Input: part model. Units: mm. Frame: model coordinates. Face numbers are marked on the shaded views. A direction names the side the tool comes from. Give positions to 0.01 mm unless a question says otherwise; leave off trailing zeros. Loops run counter-clockwise (first coordinate to the right, second up) from the corner with the lowest first, then second, coordinate; pieces in that order, holes last.
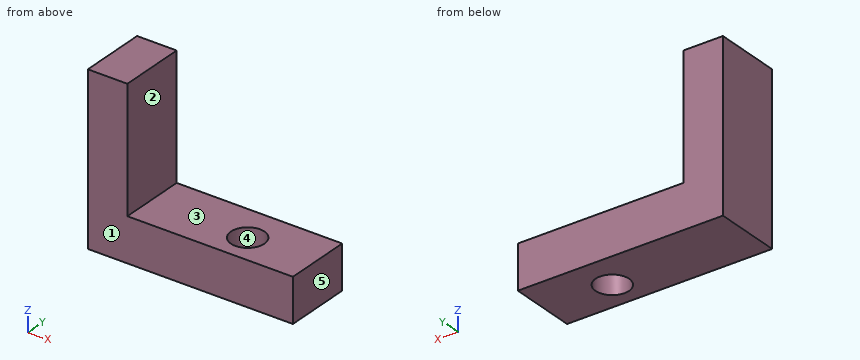
from build123d import *

# Parameters (mm, degrees)
F1_DEPTH = 25.4
F2_R     = 6.35
F3_DEPTH = 25.4


with BuildPart() as f1:
    # F0 (on Front) → F1 (new body)
    with BuildSketch(Plane.XZ):
        Polygon((-28.737951, 39.518028), (-43.749195, 39.518028), (-43.749195, -23.760144), (-28.737951, -23.760144), (34.078334, -23.760144), (34.078334, -7.132303), (-28.737951, -7.132303), align=None)
    extrude(amount=F1_DEPTH)

    # F2 (on face) → F3 (cut)
    with BuildSketch(Plane.XY.offset(-7.132303)):
        with Locations((8.678334, -14.20567)):
            Circle(F2_R)
    extrude(amount=-F3_DEPTH, mode=Mode.SUBTRACT)


solid = f1.part
(1) Ray query, probe 1 along X at (y, z) = (-23.5, -1); probe 2 along X at (y, z) = (-16, -19); probe 3 along Z at (x, y) = (-28, -21). Return the intervals inside material, ascending.
Values follow:
probe 1: x = -43.75 to -28.74
probe 2: x = -43.75 to 2.59, 14.77 to 34.08
probe 3: z = -23.76 to -7.13
(2) Cut plane D-D (y = -3.25). Return the cut outline in (x, z).
Values follow:
outline: (-43.75, -23.76) - (34.08, -23.76) - (34.08, -7.13) - (-28.74, -7.13) - (-28.74, 39.52) - (-43.75, 39.52) - close
(3) Cut plane A-A (y = -9.5). Return the cut outline in (x, z), and give its area (3 significant figures).
Values follow:
outline: (-43.75, -23.76) - (4.41, -23.76) - (4.41, -7.13) - (-28.74, -7.13) - (-28.74, 39.52) - (-43.75, 39.52) - close; (12.94, -23.76) - (34.08, -23.76) - (34.08, -7.13) - (12.94, -7.13) - close
area: 1,850 mm2
(4) Reachability of the marked faces 1 and 2 from +Z, -Z, +X, -X, +Y, -Y: full face, straight path, thin tool, end or side. Return the list, or none.
Values follow:
face 1: +Z, -Z, +X, -X, -Y
face 2: +Z, +X, +Y, -Y
(5) Pin query (flat end, axial travel): pin 1 Ø12.5 at (y, z) = (-13.5, 7) entering from +X; pin 2 Ø1.5 at (x, y) = (2, -4) entering from +Z. Return the tip coordinate at first contact, or that it passes through.
Values follow:
pin 1: stops at x = -28.74
pin 2: stops at z = -7.13
(6) Cut plane B-B (x = 12.5). Return the cut outline in (y, z), and give its area (3 significant figures).
Values follow:
outline: (-25.4, -23.76) - (-19.28, -23.76) - (-19.28, -7.13) - (-25.4, -7.13) - close; (-9.13, -23.76) - (0, -23.76) - (0, -7.13) - (-9.13, -7.13) - close
area: 254 mm2
(7) Cut plane C-C (z = -15). Return the cut outline in (x, y), and give its area (3 significant figures).
Values follow:
outline: (-43.75, -25.4) - (34.08, -25.4) - (34.08, 0) - (-43.75, 0) - close; hole circle Ø12.7 at (8.68, -14.21)
area: 1,850 mm2
(8) Mould query, pull axis X, two halves, no side actions, for the marked faces 3, 4 and 5. Classes: +X half, -X half, draft (parallel to the pull), parting line (faces both ways), or undercut.
Values follow:
face 3: draft
face 4: undercut
face 5: +X half
